Here's how the part is built. I have some questions about the finished solid (model axes, mm). A direction names the side the tool comes from. Round coordinates to 2 decimals unless told otherwise and drop trailing zeros. Write each loop counter-clockwise with the first axis right and the second up, starting at its lowest first coordinate (ties: lowest second). Pieces come first, ordered by that corner, then holes. Notation, with made-up numbers: M 56,56 L 105,56 A21 cw 105,85 Z; hole C 50.25,62 d2. An arc over 180 degrees is marked long. Use a Markdown table: item, result. Add a question column.
Solid Edge part; units mm, degrees
sketch "Sketch1" plane through (0, 0, 0) normal (0, 0, 1) x (1, 0, 0)
  line L0 (-15.5, -41) -> (-6.8711, 3.3373)
  line L1 (15.5, -41) -> (6.8711, 3.3373)
  line L2 (15.5, -45) -> (15.5, -41)
  line L3 (-8.5, -52) -> (8.5, -52)
  line L4 (-15.5, -41) -> (-15.5, -45)
  arc A0 (-6.8711, 3.3373) -> (6.8711, 3.3373) centre (0, 2) cw
  arc A1 (15.5, -45) -> (8.5, -52) centre (8.5, -45) cw
  arc A2 (-8.5, -52) -> (-15.5, -45) centre (-8.5, -45) cw
  line L5 (-2.7, -2) -> (-2.7, 2)
  line L6 (2.7, -2) -> (2.7, 2)
  arc A3 (2.7, -2) -> (-2.7, -2) centre (0, -2) cw
  arc A4 (-2.7, 2) -> (2.7, 2) centre (0, 2) cw
  arc A5 (-11.2, -41) -> (-5.8, -41) centre (-8.5, -41) cw
  line L7 (-5.8, -45) -> (-5.8, -41)
  arc A6 (-5.8, -45) -> (-11.2, -45) centre (-8.5, -45) cw
  line L8 (-11.2, -45) -> (-11.2, -41)
  arc A7 (5.8, -41) -> (11.2, -41) centre (8.5, -41) cw
  line L9 (11.2, -45) -> (11.2, -41)
  arc A8 (11.2, -45) -> (5.8, -45) centre (8.5, -45) cw
  line L10 (5.8, -45) -> (5.8, -41)
extrude "Protrusion1" add sketch "Sketch1" along normal blind 5
sketch "Sketch2" plane through (0, 0, 0) normal (1, 0, 0) x (0, 1, 0)
  line L0 (-52, 0) -> (-52, 34)
  line L1 (-52, 34) -> (-18, 34)
  line L2 (-18, 34) -> (-18, 0)
  line L3 (-18, 0) -> (-52, 0)
  dimension "D1" = 52
  dimension "D2" = 52
extrude "ExtrudedProtrusion_4" add sketch "Sketch2" along normal mid plane 6
sketch "Sketch3" plane through (0, 0, 0) normal (1, 0, 0) x (0, 1, 0)
  line L0 (-43.7, 25) -> (-43.7, 22)
  line L1 (-38.3, 25) -> (-38.3, 22)
  arc A0 (-39.0578, 26.8756) -> (-38.3, 25) centre (-41, 25) cw
  line L2 (-41, 28.8868) -> (-39.0578, 26.8756)
  line L3 (-41, 28.8868) -> (-42.9422, 26.8756)
  arc A1 (-43.7, 22) -> (-38.3, 22) centre (-41, 22) ccw
  arc A2 (-42.9422, 26.8756) -> (-43.7, 25) centre (-41, 25) ccw
  line L4 (-25.3, 25) -> (-25.3, 22)
  arc A3 (-25.3, 22) -> (-30.7, 22) centre (-28, 22) cw
  line L5 (-30.7, 25) -> (-30.7, 22)
  arc A4 (-29.9422, 26.8756) -> (-30.7, 25) centre (-28, 25) ccw
  line L6 (-28, 28.8868) -> (-29.9422, 26.8756)
  line L7 (-28, 28.8868) -> (-26.0578, 26.8756)
  arc A5 (-25.3, 25) -> (-26.0578, 26.8756) centre (-28, 25) ccw
  line L8 (-39.5, 13.5) -> (-39.5, 9.5)
  arc A6 (-39.5, 9.5) -> (-38.5, 8.5) centre (-38.5, 9.5) ccw
  line L9 (-38.5, 8.5) -> (-30.5, 8.5)
  arc A7 (-30.5, 8.5) -> (-29.5, 9.5) centre (-30.5, 9.5) ccw
  line L10 (-29.5, 9.5) -> (-29.5, 13.5)
  line L11 (-34.5, 20.6978) -> (-30.9033, 16.9733)
  line L12 (-38.0967, 16.9733) -> (-34.5, 20.6978)
  arc A8 (-39.5, 13.5) -> (-38.0967, 16.9733) centre (-34.5, 13.5) cw
  arc A9 (-29.5, 13.5) -> (-30.9033, 16.9733) centre (-34.5, 13.5) ccw
  dimension "D1" = 34.5
  dimension "D2" = 43.7
extrude "Cutout1" cut sketch "Sketch3" along normal through all and the other way through all
sketch "Sketch4" plane through (0, -23.5, 0) normal (0, -1, 0) x (1, 0, 0)
  line L0 (3, 5) -> (12.0941, 5)
  line L1 (12.0941, 5) -> (3, 14.0941)
  line L2 (3, 5) -> (3, 14.0941)
  line L3 (-3, 5) -> (-12.0941, 5)
  line L4 (-12.0941, 5) -> (-3, 14.0941)
  line L5 (-3, 14.0941) -> (-3, 5)
extrude "ExtrudedProtrusion_3" add sketch "Sketch4" along normal blind 4
fillet "Round_1" radius 10 2 edges at (0, -52, 34) (0, -18, 34)
properties material "ABS Plastic, medium impact"
Item 1: If we mould it in two halves opening along Y, with no side actions, what happens to faces 6 (the face through (15.5, -43, 2)), 7 (the face through (-13.4, -50, 2.5)), 8 (the face through (0, -27.9, 19.3))? For each: +Y half, -Y half, draft (parallel to the pull), parting line (faces both ways), or undercut.
Item 2: Imagine slicing it at A-A on x = -7.5. List the corners of the cut face in (y, z) for me, plus the area to 3 significant figures.
Item 3: Imagine slicing it at B-B on y = -20. List the corners of the cut face in (x, z) for me, plus the area to 3 significant figures.
Item 4: Imagine slicing it at C-C on y = -7. List the corners of the cut face in (x, z) for me, plus the area to 3 significant figures.
Item 5: On a 3-axis mill with a long thin cutter (end or side, diameter ignored), from which of +Z, -Z, +X, -X, +Y, -Y can I reach the whole of each face in a straight line? I mean faces 1 (the face through (-6, -23.5, 8)), 2 (the face through (-7.611, -25.472, 9.483)), 3 (the face through (0, -35, 8.5)), 4 (the face through (-0.1, 4.7, 2.5)), 5 (the face through (0, 9, 2)). Say none if no direction works.
Item 6: For pin 1 Ø5 at (x, z) = (9, 11) entering from +Y; pin 2 Ø3.5 at (x, z) = (-1, 23.5) entering from +Y; pin 3 Ø2 at (y, z) = (-35, 18.5) entering from +X; pin 4 Ø10 at (y, z) = (-44, 13) entering from +X, each with a flat end and sliding along its axis, tell me the tip position at first contact or that it passes through.
Item 7: I need wall thicknesses on probe 1 along Y at (x, z) = (-0.5, 27.5); probe 2 along Y at (x, z) = (0, 21); probe 3 along Y at (x, z) = (5, 10). Which ranges of each line are inside material? Lowest first, please. Write a range as from..to.
The answers:
| question | item | result |
|---|---|---|
| 1 | face 6 | draft |
| 1 | face 7 | -Y half |
| 1 | face 8 | undercut |
| 2 | outline | M -52,0 L -47.51,0 L -47.51,5 L -52,5 Z; M -38.49,0 L 0.11,0 L 0.11,5 L -23.5,5 L -23.5,9.59 L -27.5,9.59 L -27.5,5 L -38.49,5 Z |
| 2 | area | 234 mm² |
| 3 | outline | M -11.41,0 L 11.41,0 L 11.41,5 L 3,5 L 3,30 L -3,30 L -3,5 L -11.41,5 Z |
| 3 | area | 264 mm² |
| 4 | outline | M -8.88,0 L 8.88,0 L 8.88,5 L -8.88,5 Z |
| 4 | area | 88.8 mm² |
| 5 | face 1 | +Z, -X, +Y |
| 5 | face 2 | +Z, -X, +Y, -Y |
| 5 | face 3 | +X, -X |
| 5 | face 4 | +Z, -Z |
| 5 | face 5 | +Z, -Z, +Y |
| 6 | pin 1 | y = -23.5 |
| 6 | pin 2 | y = -18 |
| 6 | pin 3 | through |
| 6 | pin 4 | x = 3 |
| 7 | probe 1 | -51.37..-42.34, -39.66..-29.34, -26.66..-18.63 |
| 7 | probe 2 | -52..-43.51, -38.49..-30.51, -25.49..-18 |
| 7 | probe 3 | -27.5..-23.5 |
